Autodesk Inventor part; units mm, degrees
ref_plane "YZ Plane" through (0, 0, 0) normal (1, 0, 0) x (0, 1, 0)
ref_plane "XZ Plane" through (0, 0, 0) normal (0, 1, 0) x (-1, 0, 0)
ref_plane "XY Plane" through (0, 0, 0) normal (0, 0, 1) x (1, 0, 0)
sketch "Sketch1" plane through (0, 0, 0) normal (0, 1, 0) x (-1, 0, 0)
  circle A0 centre (0, 0) radius 4
  line L0 (0, 0) -> (4, 0) construction
  line L1 (0, 0) -> (0, -4) construction
  line L2 (0, 0) -> (-4, 0) construction
  line L3 (0, 0) -> (0, 4) construction
  dimension "d0" = 8
extrude "Extrusion1" add sketch "Sketch1" against normal blind 3.5
ref_plane "Work Plane1" through (0, 0, 0) normal (0, 0, 1) x (1, 0, 0)
sketch "Sketch2" plane through (0, 0, 0) normal (0, 0, 1) x (1, 0, 0)
  line L0 (-4, 0) -> (4, 0)
  line L1 (4, 0) -> (14, 0)
  line L2 (16, 0.75) -> (16, 3)
  line L3 (14.5, 3.75) -> (12.5, 3.75)
  line L4 (0, 0) -> (0, 1.25)
  line L5 (4, 0) -> (4, 1.5959) construction
  line L6 (16, 0.75) -> (14, 0.75)
  line L7 (14, 0.75) -> (14, 0)
  line L8 (16, 3) -> (14.5, 3.75)
  line L9 (12.5, 2.5) -> (12.5, 3.75)
  line L10 (5.8632, 1.8363) -> (6, 1.7244)
  line L11 (6, 1.7244) -> (6.1119, 1.8612)
  line L12 (4.1119, 1.6612) -> (4, 1.5244)
  line L13 (4, 1.5244) -> (3.8632, 1.6363)
  line L14 (1.8632, 1.4363) -> (2, 1.3244)
  line L15 (2, 1.3244) -> (2.1119, 1.4612)
  line L16 (0, 1.25) -> (1.8632, 1.4363)
  line L17 (2.1119, 1.4612) -> (3.8632, 1.6363)
  line L18 (4.1119, 1.6612) -> (5.8632, 1.8363)
  line L19 (4, 1.5244) -> (4, 3.125) construction
  line L20 (6, 1.7244) -> (6, 3.125) construction
  line L21 (6, 3.125) -> (4, 3.125) construction
  line L22 (4, 3.125) -> (2, 3.125) construction
  line L23 (2, 3.125) -> (0, 3.125) construction
  line L24 (1.8632, 1.4363) -> (2.1119, 1.4612) construction
  line L25 (3.8632, 1.6363) -> (4.1119, 1.6612) construction
  line L26 (5.8632, 1.8363) -> (6.1119, 1.8612) construction
  line L27 (1.9876, 1.4488) -> (2, 1.3244) construction
  line L28 (4, 1.65) -> (4, 1.5244) construction
  line L29 (2, 1.3244) -> (2, 3.125) construction
  line L30 (7.8632, 2.0363) -> (8, 1.9244)
  line L31 (8, 1.9244) -> (8.1119, 2.0612)
  line L32 (8, 1.9244) -> (8, 3.125) construction
  line L33 (6.1119, 1.8612) -> (7.8632, 2.0363)
  line L34 (8.1119, 2.0612) -> (12.5, 2.5)
  line L35 (8, 3.125) -> (6, 3.125) construction
  line L36 (8, 3.125) -> (12.5, 3.125) construction
  point P0 (6, 1.85)
  dimension "d8" = 16
  dimension "d11" = 14
  dimension "d12" = 0.75
  dimension "d13" = 3
  dimension "d14" = 0.75
  dimension "d15" = 1.5
  dimension "d16" = 1.25
  dimension "d19" = 3.5
  dimension "d23" = 1.25
  dimension "d25" = 0.125
  dimension "d26" = 2
  dimension "d32" = 2
revolve "Revolution1" add sketch "Sketch2" angle 360 about axis through (0, 0, 0) along (0, 1, 0)
sketch "Sketch3" plane through (0, -3.5, 0) normal (0, -1, 0) x (1, 0, 0)
  point P0 (0, 0)
  point P1 (0, 0)
sketch "Sketch4" plane through (0, -3.5, 0) normal (0, -1, 0) x (1, 0, 0)
  circle A0 centre (0, 0) radius 4
  circle A1 centre (0, 0) radius 4
  arc A2 (0, -4) -> (0, 4) centre (0, 0) ccw
  line L0 (0, 4) -> (0, -4)
extrude "Extrusion2" add sketch "Sketch4" along normal blind 2 contours A0 L0 picked at (0.5785, 1.2013)
sketch "Sketch5" plane through (0, -3.5, 0) normal (0, -1, 0) x (1, 0, 0)
  line L0 (0, -4) -> (0, 4)
  arc A0 (0, 4) -> (0, -4) centre (0, 0) ccw
extrude "Extrusion3" cut sketch "Sketch5" against normal blind 2
properties part number "Caps 8mm Square Rounded Caps Male2"
Part model, mm, in its own coordinate system. A direction names the side the tool comes from. Coordinates: 2 decimals unless noted, no trailing zeros. Write each loop counter-clockwise with the first axis right and the second up, starting at its lowest first coordinate (ties: lowest second). Pieces come first, ordered by that corner, then holes. Notation, with made-up numbers: M 62.25,22 L 99.25,22 A28 ccw 99.25,55 Z; hole C 77.5,-3.75 d1. An arc over 180 degrees is marked long. Return JSON: item names as keys, results as strings.
1. 3-axis set-ups, long thin cutter, end or side, ignore diameter. For faces 1 (the face through (-2, -1.5, 0)), 2 (the face through (3, 0, 3)), 3 (the face through (-1.82, 2.09, 8.19)): which of +Z, -Z, +X, -X, +Y, -Y reach the whole face in a straight line?
Determined:
{"face 1": "+Z, -Z, -X, -Y", "face 2": "-Y", "face 3": "+Y"}
2. Pull direction X, two halves, no side cores. Call faces 4 (the face through (11.923, 3.134, -3.755)), 5 (the face through (4, -2, 0)), 6 (the face through (0.05, 1.26, 0.1)), 7 (the face through (2, -5.5, 0)): pulls with the +X half, pulls with the -X half, needs draft (parallel to the pull), parting line crosses it, or undercut.
Determined:
{"face 4": "undercut", "face 5": "parting line crosses it", "face 6": "undercut", "face 7": "needs draft"}
3. Probe L1, parallel to Z at x = 0, y = 2.95; L2, parallel to Z at x = 0, y = 3.4; L3, parallel to X at y = 3.25, z = 0. List the from-to ranges inside material, lowest first.
Determined:
{"L1": "-16 to -12.5, 12.5 to 16", "L2": "-15.2 to -12.5, 12.5 to 15.2", "L3": "-15.5 to -12.5, 12.5 to 15.5"}
4. Flat gauge pins, fed straight in: pin 1 Ø5 at (y, z) = (-1, 6) entering from -X; pin 2 Ø4 at (x, y) = (8.5, 0.5) entering from -Z; pin 3 Ø6 at (x, z) = (-7, -4) entering from -Y; pin 4 Ø16 at (x, z) = (-3.5, 2) entering from -Y. Where does each tip first touch, or does it go through?
Determined:
{"pin 1": "x = -15.43", "pin 2": "z = -14.61", "pin 3": "y = 0", "pin 4": "y = -5.5"}
5. Saw through at B-B, the plane y = -0.75. Write the cut outline in (x, z).
Determined:
{"outline": "C 0,0 d8"}
6. Saw through at A-A, the plane y = -3.5. Write the cut outline in (x, z), then the cut area to 3 significant figures.
Determined:
{"outline": "M 0,-4 A4 ccw 0,4 Z", "area": "25.1 mm²"}
